Input: dimensioned drawing with shaded views. Units: mm. Origin: part minimum x, y, z. Round coordinates to 2 decimals unless told otherwise and drop trailing zeros. Order: outer loops, then holes, each group sorted by start corner. A loop starts at its lowest first (then second) coordinate and runs counter-clockwise, first axis right, second up. Notation, with made-up numbers: M -38.5,-13.75 L -9.5,-13.75 A12 ccw -9.5,2.25 Z; hole C -25,4 d4. An arc over 180 degrees is marked long. Use CSV: the item, a comma, the result in double quotes. Start each with the question number.
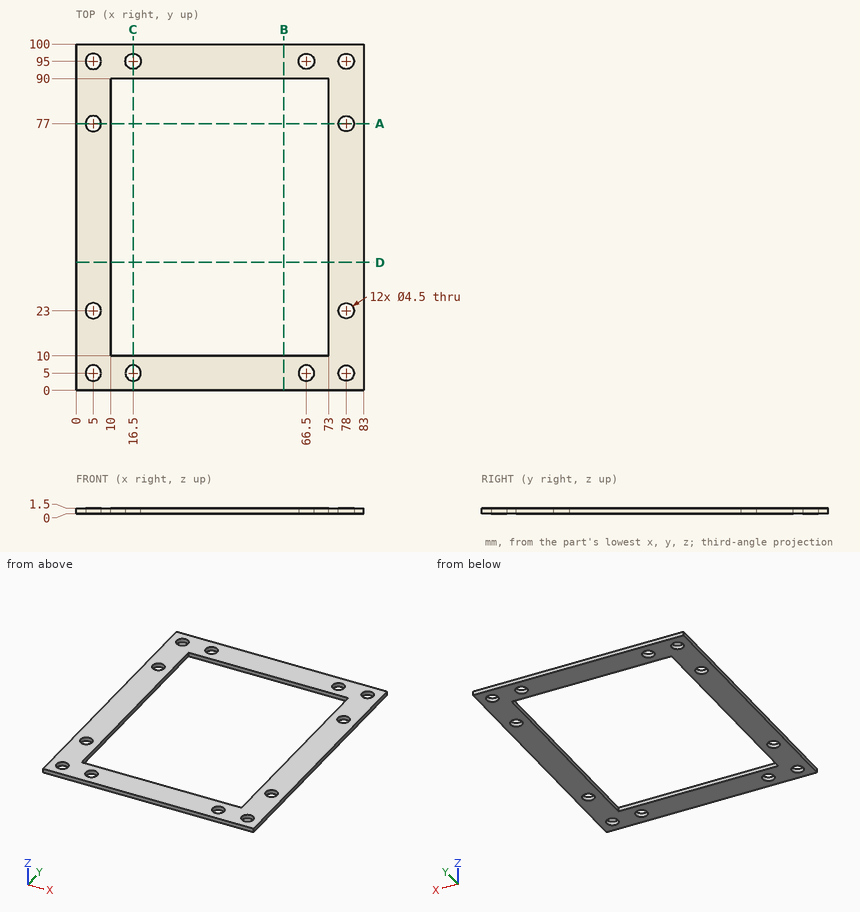
(1) Contact query for a flat-ended pin moving along its axis: P1, Ø2.5, axis at x = 16.5, y = 5, coming from the -Z side. Output: stop coordinate, or through.
(2) Section B-B on x = 60. Return loops of the section in (y, z), plus the area to 3 significant figures.
(3) Section A-A on y = 77. Return loops of the section in (x, z), plus the area to 3 significant figures.
(4) Line query: line 1 along Y through (x, z) = (66.5, 0.4); line 2 along Y through (x, z) = (5, 0.95); line 3 along Y through (x, z) = (64, 1.35). Output: solid intervals per line, ascending.
(5) Section D-D on y = 37. Return loops of the section in (x, z).
(6) Section C-C on x = 16.5. Return loops of the section in (y, z).
Results below:
1,P1,"passes through"
2,outline,"M 0,0 L 10,0 L 10,1.5 L 0,1.5 Z; M 90,0 L 100,0 L 100,1.5 L 90,1.5 Z"
2,area,"30.0 mm2"
3,outline,"M 0,0 L 2.75,0 L 2.75,1.5 L 0,1.5 Z; M 7.25,0 L 10,0 L 10,1.5 L 7.25,1.5 Z; M 73,0 L 75.75,0 L 75.75,1.5 L 73,1.5 Z; M 80.25,0 L 83,0 L 83,1.5 L 80.25,1.5 Z"
3,area,"16.5 mm2"
4,line 1,"y = 0 to 2.75, 7.25 to 10, 90 to 92.75, 97.25 to 100"
4,line 2,"y = 0 to 2.75, 7.25 to 20.75, 25.25 to 74.75, 79.25 to 92.75, 97.25 to 100"
4,line 3,"y = 0 to 10, 90 to 100"
5,outline,"M 0,0 L 10,0 L 10,1.5 L 0,1.5 Z; M 73,0 L 83,0 L 83,1.5 L 73,1.5 Z"
6,outline,"M 0,0 L 2.75,0 L 2.75,1.5 L 0,1.5 Z; M 7.25,0 L 10,0 L 10,1.5 L 7.25,1.5 Z; M 90,0 L 92.75,0 L 92.75,1.5 L 90,1.5 Z; M 97.25,0 L 100,0 L 100,1.5 L 97.25,1.5 Z"
